```python
from build123d import *

# Parameters (mm, degrees)
SALIENTE_EXTRUIR2_DEPTH                              = 10
REDONDEO3_R                                          = 15
REDONDEO5_R                                          = 50
CROQUIS4_R                                           = 2.8
CROQUIS4_R_2                                         = 2.25
CORTAR_EXTRUIR1_DEPTH                                = 149.996644258
REFRENTADO_PARA_TORNILLO_CON_CABEZA_TRON_D           = 4.5
REFRENTADO_PARA_TORNILLO_CON_CABEZA_TRON_CBORE_D     = 7.5
REFRENTADO_PARA_TORNILLO_CON_CABEZA_TRON_CBORE_DEPTH = 5
CORTAR_EXTRUIR2_DEPTH                                = 6


with BuildPart() as part:
    # Croquis2 → Saliente-Extruir2 (new body)
    with BuildSketch(Plane(origin=(0, 0, 0), x_dir=(0, 1, 0), z_dir=(0, 0, 1))):
        with BuildLine():
            Line((-85, 52.678268764), (-85, 110))
            Line((-85, 110), (85, 110))
            Line((85, 110), (85, 52.678268764))
            ThreePointArc((85, 52.678268764), (0, -100), (-85, 52.678268764))
        make_face()
    extrude(amount=SALIENTE_EXTRUIR2_DEPTH)

    # Redondeo3
    redondeo3_edges = [part.edges().sort_by_distance(p)[0] for p in [
        (-110, -85, 5),
        (-110, 85, 5),
    ]]
    fillet(redondeo3_edges, radius=REDONDEO3_R)

    # Redondeo5
    redondeo5_edges = [part.edges().sort_by_distance(p)[0] for p in [
        (-52.678268764, 85, 5),
        (-52.678268764, -85, 5),
    ]]
    fillet(redondeo5_edges, radius=REDONDEO5_R)

    # Croquis4 → Cortar-Extruir1 (cut, through all)
    with BuildSketch(Plane.XY.offset(10)):
        with Locations((-93, 69.2)):
            Circle(CROQUIS4_R)
        with Locations((-93, 52.279001067)):
            Circle(CROQUIS4_R)
        with Locations((-93, -52.279001068)):
            Circle(CROQUIS4_R)
        with Locations((-93, -69.2)):
            Circle(CROQUIS4_R)
        with Locations((-13, 39)):
            Circle(CROQUIS4_R_2)
        with Locations((43, 39)):
            Circle(CROQUIS4_R_2)
        with Locations((-13, 65)):
            Circle(CROQUIS4_R_2)
        with Locations((43, 65)):
            Circle(CROQUIS4_R_2)
        with Locations((-13, -62)):
            Circle(CROQUIS4_R_2)
        with Locations((43, -62)):
            Circle(CROQUIS4_R_2)
        with BuildLine():
            Line((-58.219532094, 11.25), (-70.219532094, 11.25))
            ThreePointArc((-70.219532094, 11.25), (-72.469532094, 13.5), (-70.219532094, 15.75))
            Line((-70.219532094, 15.75), (-58.219532094, 15.75))
            ThreePointArc((-58.219532094, 15.75), (-55.969532094, 13.5), (-58.219532094, 11.25))
        make_face()
        with BuildLine():
            Line((-33.219532094, 11.25), (-45.219532094, 11.25))
            ThreePointArc((-45.219532094, 11.25), (-47.469532094, 13.5), (-45.219532094, 15.75))
            Line((-45.219532094, 15.75), (-33.219532094, 15.75))
            ThreePointArc((-33.219532094, 15.75), (-30.969532094, 13.5), (-33.219532094, 11.25))
        make_face()
        with BuildLine():
            Line((-58.219532094, -26.75), (-70.219532094, -26.75))
            ThreePointArc((-70.219532094, -26.75), (-72.469532094, -24.5), (-70.219532094, -22.25))
            Line((-70.219532094, -22.25), (-58.219532094, -22.25))
            ThreePointArc((-58.219532094, -22.25), (-55.969532094, -24.5), (-58.219532094, -26.75))
        make_face()
    extrude(amount=-CORTAR_EXTRUIR1_DEPTH, mode=Mode.SUBTRACT)

    # Refrentado para tornillo con cabeza tron (through all)
    with Locations(Plane.XY.offset(10)):
        with Locations((-80, 0), (80, 0)):
            CounterBoreHole(REFRENTADO_PARA_TORNILLO_CON_CABEZA_TRON_D / 2, REFRENTADO_PARA_TORNILLO_CON_CABEZA_TRON_CBORE_D / 2, REFRENTADO_PARA_TORNILLO_CON_CABEZA_TRON_CBORE_DEPTH)

    # Croquis7 → Cortar-Extruir2 (cut)
    with BuildSketch(Plane(origin=(0, 0, 0), x_dir=(1, 0, 0), z_dir=(0, 0, -1))):
        with BuildLine():
            Line((-70.219532094, 29), (-58.219532094, 29))
            ThreePointArc((-58.219532094, 29), (-53.719532094, 24.5), (-58.219532094, 20))
            Line((-58.219532094, 20), (-70.219532094, 20))
            ThreePointArc((-70.219532094, 20), (-74.719532094, 24.5), (-70.219532094, 29))
        make_face()
        with BuildLine():
            Line((-70.219532094, -9), (-58.219532094, -9))
            ThreePointArc((-58.219532094, -9), (-53.719532094, -13.5), (-58.219532094, -18))
            Line((-58.219532094, -18), (-70.219532094, -18))
            ThreePointArc((-70.219532094, -18), (-74.719532094, -13.5), (-70.219532094, -9))
        make_face()
        with BuildLine():
            Line((-45.219532094, -9), (-33.219532094, -9))
            ThreePointArc((-33.219532094, -9), (-28.719532094, -13.5), (-33.219532094, -18))
            Line((-33.219532094, -18), (-45.219532094, -18))
            ThreePointArc((-45.219532094, -18), (-49.719532094, -13.5), (-45.219532094, -9))
        make_face()
    extrude(amount=-CORTAR_EXTRUIR2_DEPTH, mode=Mode.SUBTRACT)


solid = part.part
```
Geometry check sheet. Reference: the model listing, model coordinates, mm. A direction names the side the tool comes from. Round coordinates to 2 decimals unless told otherwise and drop trailing zeros. Loops run counter-clockwise (first coordinate to the right, second up) from the corner with the lowest first, then second, coordinate; pieces in that order, holes last. Notation, with made-up numbers: (12, 66) - (59, 66) arc R25 cw to (59, 94) - close; hole circle Ø7 at (-37, 4). An arc over 180 degrees is marked (long way). Use a Markdown table: item, result.
Q1. Draft check along Y on faces 4 (the flat face through (-80, 85, 5)), 5 (the cylindrical face through (-105.49, -80.72, 5.07)), 6 (the cylindrical face through (-53.72, 13.4, 2.96)). Enter one of: released by +Y, released by -Y, zero draft, split by the parting line, or undercut.
Solutions:
| item | result |
|---|---|
| face 4 | released by +Y |
| face 5 | released by -Y |
| face 6 | undercut |
Q2. Material ranges on line 1 (Y direction, x = -93, z = 6.25); line 2 (Y direction, x = -66, z = 0.5); line 3 (Y direction, x = -1, z = 8.5) (3 decimals), recorded low to high.
Solutions:
| item | result |
|---|---|
| line 1 | y = -85 to -72, -66.4 to -55.08, -49.48 to 49.48, 55.08 to 66.4, 72 to 85 |
| line 2 | y = -85 to -29, -20 to 9, 18 to 85 |
| line 3 | y = -99.995 to 99.995 |
Q3. Go/stop test with flat-tipped pins: P1, Ø2, axis at x = -62.5, z = 8, coming from the -Y side; P2, Ø4, axis at x = -64, z = 5.5, coming from the -Y side; P3, Ø8, axis at x = -82, y = -0.5, coming from the +Z side; P4, Ø4.5, axis at x = -64, y = -22.5, coming from the -Z side. Record where each tip stops, or that it passes through.
Solutions:
| item | result |
|---|---|
| P1 | stops at y = -85.15 |
| P2 | stops at y = -85.11 |
| P3 | stops at z = 10 |
| P4 | stops at z = 6 |
Q4. Cross-section at B-B on x = 50. Record the cut outline in (y, z).
Solutions:
| item | result |
|---|---|
| outline | (-86.6, 0) - (86.6, 0) - (86.6, 10) - (-86.6, 10) - close |
Q5. Cross-section at A-A on y = -38.5. Record the cut outline in (x, z).
Solutions:
| item | result |
|---|---|
| outline | (-110, 0) - (92.29, 0) - (92.29, 10) - (-110, 10) - close |
Q6. Access from +Z, -Z, +X, -X, +Y, -Y to the whole of each face (thin tool, end or side, straight path). Record for faces 1 (the cylindrical face through (-74.72, -24.4, 2.96)), 2 (the cylindrical face through (-91.49, 71.56, 5.07)), 3 (the cylindrical face through (-76.536, -1.436, 7.535)).
Solutions:
| item | result |
|---|---|
| face 1 | -Z |
| face 2 | +Z, -Z |
| face 3 | +Z |
